from build123d import *

# Parameters (mm, degrees)
SKETCH1_W            = 145.4
SKETCH1_H            = 52.4
BOSS_EXTRUDE1_DEPTH  = 27.2
SKETCH2_W            = 140.4
SKETCH2_H            = 47.4
CUT_EXTRUDE1_DEPTH   = 25.2
SKETCH3_W            = 46.4
SKETCH3_H            = 25.2
CUT_EXTRUDE2_DEPTH   = 25.2
SKETCH4_W            = 6
SKETCH4_H            = 6
BOSS_EXTRUDE2_DEPTH  = 4
FILLET1_R            = 2
FILLET2_R            = 2
SKETCH7_R            = 1.5
CUT_EXTRUDE4_DEPTH   = 4
SKETCH8_W            = 2.5
SKETCH8_H            = 52.4
CUT_EXTRUDE5_DEPTH   = 43
SKETCH9_W            = 47.4
SKETCH9_H            = 21.2
CUT_EXTRUDE6_DEPTH   = 43
SKETCH11_W           = 137.9
SKETCH11_H           = 17.288060203
CUT_EXTRUDE7_DEPTH   = 59
SKETCH12_W           = 134.4
SKETCH12_H           = 44.280487354
CUT_EXTRUDE8_DEPTH   = 10
SKETCH16_W           = 12
SKETCH16_H           = 2.5
BOSS_EXTRUDE4_DEPTH  = 8
FILLET3_R            = 2
SKETCH17_R           = 1
BOSS_EXTRUDE5_DEPTH  = 5
SKETCH18_W           = 12
SKETCH18_H           = 2.5
BOSS_EXTRUDE6_DEPTH  = 8
FILLET4_R            = 2
SKETCH19_R           = 1
BOSS_EXTRUDE7_DEPTH  = 10
SKETCH20_W           = 12
SKETCH20_H           = 2.5
BOSS_EXTRUDE8_DEPTH  = 8
FILLET5_R            = 2
SKETCH21_R           = 1
BOSS_EXTRUDE9_DEPTH  = 5
SKETCH22_W           = 12
SKETCH22_H           = 2.5
BOSS_EXTRUDE10_DEPTH = 8
FILLET6_R            = 2
SKETCH23_R           = 1
BOSS_EXTRUDE11_DEPTH = 5


with BuildPart() as part:
    # Sketch1 → Boss-Extrude1 (new body)
    with BuildSketch(Plane(origin=(0, 0, 0), x_dir=(1, 0, 0), z_dir=(0, 1, 0))):
        Rectangle(SKETCH1_W, SKETCH1_H)
    extrude(amount=BOSS_EXTRUDE1_DEPTH)

    # Sketch2 → Cut-Extrude1 (cut)
    with BuildSketch(Plane(origin=(0, 27.2, 0), x_dir=(1, 0, 0), z_dir=(0, 1, 0))):
        Rectangle(SKETCH2_W, SKETCH2_H)
    extrude(amount=-CUT_EXTRUDE1_DEPTH, mode=Mode.SUBTRACT)

    # Sketch3 → Cut-Extrude2 (cut)
    with BuildSketch(Plane.ZY.offset(-70.2)):
        with Locations((0.5, 14.6)):
            Rectangle(SKETCH3_W, SKETCH3_H)
    extrude(amount=-CUT_EXTRUDE2_DEPTH, mode=Mode.SUBTRACT)

    # Sketch4 → Boss-Extrude2 (add)
    with BuildSketch(Plane(origin=(0, 27.2, 0), x_dir=(1, 0, 0), z_dir=(0, 1, 0))):
        with Locations((3, -29.2)):
            Rectangle(SKETCH4_W, SKETCH4_H)
        with Locations((3, 29.2)):
            Rectangle(SKETCH4_W, SKETCH4_H)
    extrude(amount=-BOSS_EXTRUDE2_DEPTH)

    # Fillet1
    fillet1_edges = [part.edges().sort_by_distance(p)[0] for p in [
        (0, 25.2, -32.2),
        (6, 25.2, -32.2),
    ]]
    fillet(fillet1_edges, radius=FILLET1_R)

    # Fillet2
    fillet2_edges = [part.edges().sort_by_distance(p)[0] for p in [
        (0, 25.2, 32.2),
        (6, 25.2, 32.2),
    ]]
    fillet(fillet2_edges, radius=FILLET2_R)

    # Sketch7 → Cut-Extrude4 (cut)
    with BuildSketch(Plane(origin=(0, 23.2, 0), x_dir=(-1, 0, 0), z_dir=(0, -1, 0))):
        with Locations(Location((-3, -29.2, 0), (0, 0, 90))):
            Circle(SKETCH7_R)
        with Locations(Location((-3, 29.2, 0), (0, 0, 90))):
            Circle(SKETCH7_R)
    extrude(amount=-CUT_EXTRUDE4_DEPTH, mode=Mode.SUBTRACT)

    # Sketch8 → Cut-Extrude5 (cut)
    with BuildSketch(Plane(origin=(0, 27.2, 0), x_dir=(1, 0, 0), z_dir=(0, 1, 0))):
        with Locations((71.45, 0)):
            Rectangle(SKETCH8_W, SKETCH8_H)
    extrude(amount=-CUT_EXTRUDE5_DEPTH, mode=Mode.SUBTRACT)

    # Sketch9 → Cut-Extrude6 (cut)
    with BuildSketch(Plane.ZY.offset(72.7)):
        with Locations((0, 13.6)):
            Rectangle(SKETCH9_W, SKETCH9_H)
    extrude(amount=-CUT_EXTRUDE6_DEPTH, mode=Mode.SUBTRACT)

    # Sketch11 → Cut-Extrude7 (cut)
    with BuildSketch(Plane(origin=(0, 0, -26.2), x_dir=(-1, 0, 0), z_dir=(0, 0, -1))):
        with Locations((1.25, 13.644030102)):
            Rectangle(SKETCH11_W, SKETCH11_H)
    extrude(amount=-CUT_EXTRUDE7_DEPTH, mode=Mode.SUBTRACT)

    # Sketch12 → Cut-Extrude8 (cut)
    with BuildSketch(Plane(origin=(0, 0, 0), x_dir=(-1, 0, 0), z_dir=(0, -1, 0))):
        Rectangle(SKETCH12_W, SKETCH12_H)
    extrude(amount=-CUT_EXTRUDE8_DEPTH, mode=Mode.SUBTRACT)

    # Sketch16 → Boss-Extrude4 (add)
    with BuildSketch(Plane(origin=(0, 0, -26.2), x_dir=(-1, 0, 0), z_dir=(0, 0, -1))):
        with Locations((-64.2, 25.95)):
            Rectangle(SKETCH16_W, SKETCH16_H)
    extrude(amount=BOSS_EXTRUDE4_DEPTH)

    # Fillet3
    fillet3_edges = [part.edges().sort_by_distance(p)[0] for p in [
        (70.2, 25.95, -34.2),
        (58.2, 25.95, -34.2),
    ]]
    fillet(fillet3_edges, radius=FILLET3_R)

    # Sketch17 → Boss-Extrude5 (add)
    with BuildSketch(Plane(origin=(0, 24.7, 0), x_dir=(-1, 0, 0), z_dir=(0, -1, 0))):
        with Locations(Location((-67.2, 31.2, 0), (0, 0, 270))):
            Circle(SKETCH17_R)
        with Locations(Location((-61.2, 31.2, 0), (0, 0, 270))):
            Circle(SKETCH17_R)
    extrude(amount=BOSS_EXTRUDE5_DEPTH)

    # Sketch18 → Boss-Extrude6 (add)
    with BuildSketch(Plane.XY.offset(26.2)):
        with Locations((64.2, 25.95)):
            Rectangle(SKETCH18_W, SKETCH18_H)
    extrude(amount=BOSS_EXTRUDE6_DEPTH)

    # Fillet4
    fillet4_edges = [part.edges().sort_by_distance(p)[0] for p in [
        (70.2, 25.95, 34.2),
        (58.2, 25.95, 34.2),
    ]]
    fillet(fillet4_edges, radius=FILLET4_R)

    # Sketch19 → Boss-Extrude7 (add)
    with BuildSketch(Plane(origin=(0, 24.7, 0), x_dir=(-1, 0, 0), z_dir=(0, -1, 0))):
        with Locations(Location((-67.2, -31.2, 0), (0, 0, 270))):
            Circle(SKETCH19_R)
        with Locations(Location((-61.2, -31.2, 0), (0, 0, 270))):
            Circle(SKETCH19_R)
    extrude(amount=BOSS_EXTRUDE7_DEPTH)

    # Sketch20 → Boss-Extrude8 (add)
    with BuildSketch(Plane.XY.offset(26.2)):
        with Locations((-66.7, 25.95)):
            Rectangle(SKETCH20_W, SKETCH20_H)
    extrude(amount=BOSS_EXTRUDE8_DEPTH)

    # Fillet5
    fillet5_edges = [part.edges().sort_by_distance(p)[0] for p in [
        (-72.7, 25.95, 34.2),
        (-60.7, 25.95, 34.2),
    ]]
    fillet(fillet5_edges, radius=FILLET5_R)

    # Sketch21 → Boss-Extrude9 (add)
    with BuildSketch(Plane(origin=(0, 24.7, 0), x_dir=(-1, 0, 0), z_dir=(0, -1, 0))):
        with Locations(Location((63.7, -31.2, 0), (0, 0, 270))):
            Circle(SKETCH21_R)
        with Locations(Location((69.7, -31.2, 0), (0, 0, 270))):
            Circle(SKETCH21_R)
    extrude(amount=BOSS_EXTRUDE9_DEPTH)

    # Sketch22 → Boss-Extrude10 (add)
    with BuildSketch(Plane(origin=(0, 0, -26.2), x_dir=(-1, 0, 0), z_dir=(0, 0, -1))):
        with Locations((66.7, 25.95)):
            Rectangle(SKETCH22_W, SKETCH22_H)
    extrude(amount=BOSS_EXTRUDE10_DEPTH)

    # Fillet6
    fillet6_edges = [part.edges().sort_by_distance(p)[0] for p in [
        (-72.7, 25.95, -34.2),
        (-60.7, 25.95, -34.2),
    ]]
    fillet(fillet6_edges, radius=FILLET6_R)

    # Sketch23 → Boss-Extrude11 (add)
    with BuildSketch(Plane(origin=(0, 24.7, 0), x_dir=(-1, 0, 0), z_dir=(0, -1, 0))):
        with Locations(Location((63.7, 31.2, 0), (0, 0, 270))):
            Circle(SKETCH23_R)
        with Locations(Location((69.7, 31.2, 0), (0, 0, 270))):
            Circle(SKETCH23_R)
    extrude(amount=BOSS_EXTRUDE11_DEPTH)


solid = part.part
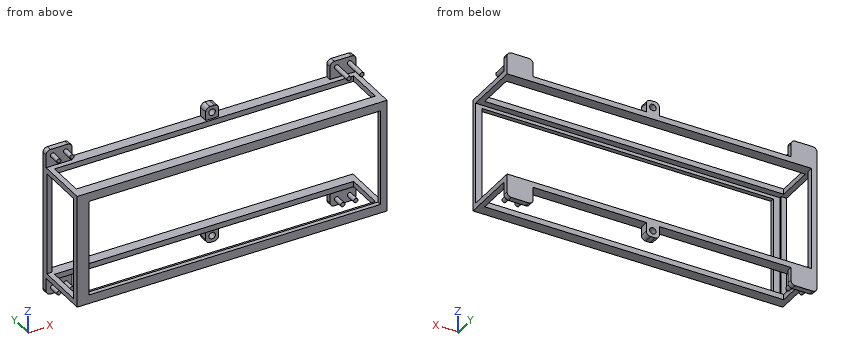
Read the model definition and answer for the solid it produces. Units are mm, in the model's axes. Coordinates: 2 decimals unless noted, no trailing zeros. Loops run counter-clockwise (first coordinate to the right, second up) from the corner with the lowest first, then second, coordinate; pieces in that order, holes last. Notation, with made-up numbers: (17, -15.5) - (25, -15.5) arc R14 ccw to (25, 0.5) - close; hole circle Ø9 at (45.5, 49.25). An arc over 180 degrees is marked (long way). Answer in a Markdown table with one row per item.
Q1. Straight lines are drawn through the part: line 1 along X through (y, z) = (24.9, -29.2); line 2 along X through (y, z) = (24.2, 29.2); line 3 along Z through (x, y) = (27.5, 26). For each, find the intervals that lie inside material, in ascending order. Write a range as [from, to].
Here are the results:
| item | result |
|---|---|
| line 1 | x = [-72.7, -60.7], [0, 1.5], [4.5, 6], [58.2, 70.2] |
| line 2 | x = [0, 1.5], [4.5, 6] |
| line 3 | z = [-26.2, -23.7], [23.7, 26.2] |
Q2. Find section B-B on z = -20.5. Write down the section's boundary in (x, y).
Here are the results:
| item | result |
|---|---|
| outline | (-72.7, 0) - (-67.2, 0) - (-67.2, 2) - (-70.2, 2) - (-70.2, 3) - (-72.7, 3) - close; (-72.7, 24.2) - (-70.2, 24.2) - (-70.2, 27.2) - (-72.7, 27.2) - close; (67.2, 0) - (70.2, 0) - (70.2, 2) - (67.2, 2) - close |
Q3. Given P1, Ø1.6, axis at x = 67, z = -31, coming from the -Y side; P2, Ø1.6, axis at x = 24, y = 1, coming from the +Z side; P3, Ø3, axis at x = 4.5, z = 30, coming from the -Y side, each flat-ended and moving along its own axis, determine where each tip first touches the part or whether it passes through.
Here are the results:
| item | result |
|---|---|
| P1 | stops at y = 19.7 |
| P2 | stops at z = 26.2 |
| P3 | stops at y = 23.2 |
Q4. Find section A-A on x = -32.5. Write down the section's boundary in (y, z).
Here are the results:
| item | result |
|---|---|
| outline | (0, -26.2) - (5, -26.2) - (5, -23.7) - (2, -23.7) - (2, -22.14) - (0, -22.14) - close; (0, 22.14) - (2, 22.14) - (2, 23.7) - (5, 23.7) - (5, 26.2) - (0, 26.2) - close; (22.29, -26.2) - (27.2, -26.2) - (27.2, -23.7) - (22.29, -23.7) - close; (22.29, 23.7) - (27.2, 23.7) - (27.2, 26.2) - (22.29, 26.2) - close |
Q5. Find section C-C on y = 9. Write down the section's boundary in (x, z).
Here are the results:
| item | result |
|---|---|
| outline | (-72.7, -26.2) - (-70.2, -26.2) - (-70.2, -23.7) - (-72.7, -23.7) - close; (-72.7, 23.7) - (-70.2, 23.7) - (-70.2, 26.2) - (-72.7, 26.2) - close; (67.7, -26.2) - (70.2, -26.2) - (70.2, -23.7) - (67.7, -23.7) - close; (67.7, 23.7) - (70.2, 23.7) - (70.2, 26.2) - (67.7, 26.2) - close |
